Autodesk Inventor part; units mm, degrees
ref_plane "YZ Plane" through (0, 0, 0) normal (1, 0, 0) x (0, 1, 0)
ref_plane "XZ Plane" through (0, 0, 0) normal (0, 1, 0) x (-1, 0, 0)
ref_plane "XY Plane" through (0, 0, 0) normal (0, 0, 1) x (1, 0, 0)
sketch "Sketch1" plane through (0, 0, 0) normal (0, 1, 0) x (-1, 0, 0)
  line L0 (0, 0) -> (-12.7, 0)
  line L1 (-12.7, 0) -> (-12.7, 50.8)
  line L2 (-12.7, 50.8) -> (0, 50.8)
  line L3 (0, 50.8) -> (0, 0)
  circle A0 centre (-6.35, 3.175) radius 4.7625
  point P0 (-1.5875, 0)
  point P1 (-11.1125, 0)
  dimension "d1" = 12.7
  dimension "d4" = 50.8
  dimension "d11" = 9.525
  dimension "d12" = 3.175
  dimension "d13" = 6.35
extrude "Extrusion1" add sketch "Sketch1" along normal blind 0.3175 contours L0 A0 L1 L2 L3 | L0 A0 picked at (-5.1617, 2.7426)
sketch "Sketch2" plane through (0, 0.3175, 0) normal (0, 1, 0) x (1, 0, 0)
  line L0 (11.1125, -49.2125) -> (11.1125, -39.6875) construction
  line L1 (12.7, -49.2125) -> (12.7, -39.6875)
  line L2 (9.525, -39.6875) -> (9.525, -49.2125)
  arc A0 (9.525, -49.2125) -> (12.7, -49.2125) centre (11.1125, -49.2125) ccw
  arc A1 (12.7, -39.6875) -> (9.525, -39.6875) centre (11.1125, -39.6875) ccw
  line L3 (0, -50.8) -> (12.7, -50.8)
  point P0 (0, 0)
  point P1 (11.1125, -44.45)
  dimension "d23" = 1.5875
  dimension "d24" = 1.5875
  dimension "d25" = 9.525
extrude "Extrusion2" add sketch "Sketch2" along normal blind 12.7
sketch "Sketch3" plane through (0, 0.3175, 0) normal (0, 1, 0) x (1, 0, 0)
  line L0 (12.7, -50.8) -> (0, -50.8)
  line L1 (12.7, 0) -> (12.7, -50.8)
  line L2 (11.1125, -50.8) -> (12.7, -50.8)
  line L3 (12.7, -50.8) -> (12.7, -49.2125)
  arc A0 (11.1125, -50.8) -> (12.7, -49.2125) centre (11.1125, -49.2125) ccw
  point P0 (0, 0)
extrude "Extrusion3" cut sketch "Sketch3" against normal blind 12.7
sketch "Sketch4" plane through (0, 0.3175, 0) normal (0, 1, 0) x (1, 0, 0)
  circle A0 centre (6.35, -3.175) radius 4.7625
  line L0 (12.7, -39.6875) -> (12.7, 0)
  line L1 (12.7, 0) -> (0, 0)
  dimension "d14" = 9.525
  dimension "d15" = 6.35
  dimension "d16" = 3.175
extrude "Extrusion4" cut sketch "Sketch4" against normal blind 12.7
sketch "Sketch5" plane through (0, 0.3175, 0) normal (0, 1, 0) x (1, 0, 0)
  line L0 (0, -3.175) -> (1.5875, 0)
  line L1 (2.8002, 0) -> (0, 0)
  line L2 (0, -50.8) -> (0, 0)
  line L3 (0, -3.175) -> (0, 0)
  line L4 (0, 0) -> (1.5875, 0)
extrude "Extrusion5" cut sketch "Sketch5" against normal blind 12.7
sketch "Sketch6" plane through (0, 0.3175, 0) normal (0, 1, 0) x (1, 0, 0)
  line L0 (11.2433, 0) -> (12.7, -3.175)
  line L1 (12.7, -39.6875) -> (12.7, 0)
  line L2 (12.7, -3.175) -> (12.7, 0)
  line L3 (12.7, 0) -> (11.2433, 0)
  line L4 (12.7, 0) -> (9.8998, 0)
  point P0 (0, 0)
extrude "Extrusion6" cut sketch "Sketch6" against normal blind 12.7
properties part number "piston locking tool"
The model under review builds one solid part; all positions refer to its coordinate system, in mm. A direction names the side the tool comes from. Coordinates: 2 decimals unless noted, no trailing zeros. Write each loop counter-clockwise with the first axis right and the second up, starting at its lowest first coordinate (ties: lowest second). Pieces come first, ordered by that corner, then holes. Notation, with made-up numbers: (13.25, 70.5) - (41.25, 70.5) arc R24 ccw to (41.25, 92.5) - close; hole circle Ø2 at (-33.5, 49.5). An arc over 180 degrees is marked (long way). Write item = value, one per line.
(1) Consider section C-C, the plane x = 12. Give the boundary of the cut face in (y, z), then the cut area to 3 significant figures.
Result sheet:
outline = (0, 1.65) - (0.32, 1.65) - (0.32, 38.37) - (13.02, 38.37) - (13.02, 50.53) - (0, 50.53) - close
area = 170 mm^2
(2) Consider section A-A, the plane y = 4.5. Give the boundary of the cut face in (x, z) (1 decimal), then the cut area to 3 significant figures.
Result sheet:
outline = (9.5, 39.7) arc R1.6 ccw to (12.7, 39.7) - (12.7, 49.2) arc R1.6 ccw to (9.5, 49.2) - close
area = 38.2 mm^2
(3) For P1, Ø3, axis at y = 6, z = 37, coming from the +X side, flat-tipped, find the tip position at first contact; note if it passes through.
Result sheet:
P1 = 12.17
(4) For line 1 (Z direction, x = 6.35, y = 0.2); line 2 (Y direction, x = 6, z = 31.5); line 3 (X direction, y = 11.25, z = 48) (3 decimals), list the stretches that pass through material, from the lowest coordinate up. Write a range as [from, to].
Result sheet:
line_1 = [7.94, 50.8]
line_2 = [0, 0.32]
line_3 = [9.525, 12.7]
(5) Machinability: for faces 1 (the face through (11.1, 6.4, 50.8)), 2 (the face through (11.1, 6.6, 38.1)), 3 (the face through (9.525, 7, 44)), which of the approach directions +Z, -Z, +X, -X, +Y, -Y give a long, thin tool a straight path to every point of the face, cutting with its end or side? Answer none if there is none.
Result sheet:
face_1 = +Z, +Y
face_2 = -Z, +Y
face_3 = +Z, -Z, -X, +Y
(6) Consider section B-B, the plane x = 6.35. Give the boundary of the cut face in (y, z), then the cut area to 3 significant figures.
Result sheet:
outline = (0, 7.94) - (0.32, 7.94) - (0.32, 50.8) - (0, 50.8) - close
area = 13.6 mm^2
